Could you check a few things on this model? Use its own coordinates, in mm. Face numbers are marked on the shaded views. A direction names the side the tool comes from. Give positions to 0.01 mm unless a question says otherwise; leave off trailing zeros. Loops run counter-clockwise (first coordinate to the right, second up) from the corner with the lowest first, then second, coordinate; pieces in that order, holes last. Notation, with made-up numbers: (19.5, -4) - (35.5, -4) arc R14 cw to (35.5, 23) - close; hole circle Ø9 at (-12, 76.25). An arc over 180 degrees is marked (long way). Write each question's results on one line, items separated by ' | '. Start each with the question number.
1) I want a section at D-D, the plane z = 0. Write out the boundary of the cut face in (x, y), and give its area (3 significant figures).
2) On a 3-axis mill with a long thin cutter (end or side, diameter ignored), from which of +Z, -Z, +X, -X, +Y, -Y can I reach the whole of each face in a straight line? I mean the marked faces 4, 5 and 6. Say none if no direction works.
3) I'm going to push flat-ended pins straight in: pin 1 (5.5 mm diameter, centred on y = 53, z = -11, fed in from -X); pin 2 (1.5 mm diameter, centred on y = 7.5, z = -11.5, fed in from +X); pin 3 (6 mm diameter, centred on y = 36.5, z = -9.5, fed in from +X); pin 4 (3 mm diameter, centred on x = 0, z = 0, fed in from +Y). Where does each tip first touch, or does it pass through?
4) I want a section at B-B, the plane y = 5.5. Write out the boundary of the cut face in (x, z).
5) If I drill on probe 1 along X at (y, z) = (2.1, 0); probe 2 along Z at (x, y) = (-5, 30.5); probe 3 along Y at (x, z) = (-7, 8.5), over which ranges is the centre line in solid material (lowest first)? Write a range as [from, to].
6) I want a section at C-C, the plane x = -1.5. Write out the boundary of the cut face in (y, z), and give its area (3 significant figures).
7) If we mould it in two halves opening along Z, with no side actions, what happens to the marked faces 1, 2 and 3? For each: +Z half, -Z half, draft (parallel to the pull), parting line (faces both ways), or undercut.
8) I want a section at A-A, the plane z = 6. Write out the boundary of the cut face in (x, y).
from build123d import *

# Parameters (mm, degrees)
SKETCH1_W           = 40
SKETCH1_H           = 26
BOSS_EXTRUDE1_DEPTH = 3
SKETCH2_R           = 1.75
CUT_EXTRUDE1_DEPTH  = 3
SKETCH3_W           = 19.25
SKETCH3_H           = 3
BOSS_EXTRUDE2_DEPTH = 56.5
SKETCH5_W           = 19.25
SKETCH5_H           = 5
BOSS_EXTRUDE4_DEPTH = 12
SKETCH6_R           = 2.5
CUT_EXTRUDE2_DEPTH  = 15
SKETCH7_W           = 26
SKETCH7_H           = 60
BOSS_EXTRUDE5_DEPTH = 4


with BuildPart() as part:
    # Sketch1 → Boss-Extrude1 (new body)
    with BuildSketch(Plane(origin=(0, 0, 0), x_dir=(1, 0, 0), z_dir=(0, 1, 0))):
        Rectangle(SKETCH1_W, SKETCH1_H)
    extrude(amount=BOSS_EXTRUDE1_DEPTH)

    # Sketch2 → Cut-Extrude1 (cut)
    with BuildSketch(Plane(origin=(0, 3, 0), x_dir=(1, 0, 0), z_dir=(0, 1, 0))):
        with Locations(Location((14.3, 0, 0), (0, 0, 270))):
            Circle(SKETCH2_R)
        with Locations(Location((-14.3, 0, 0), (0, 0, 90))):
            Circle(SKETCH2_R)
    extrude(amount=-CUT_EXTRUDE1_DEPTH, mode=Mode.SUBTRACT)

    # Sketch3 → Boss-Extrude2 (add)
    with BuildSketch(Plane(origin=(0, 3, 0), x_dir=(1, 0, 0), z_dir=(0, 1, 0))):
        with Locations((0.625, -11.5)):
            Rectangle(SKETCH3_W, SKETCH3_H)
        with Locations((0.625, 11.5)):
            Rectangle(SKETCH3_W, SKETCH3_H)
    extrude(amount=BOSS_EXTRUDE2_DEPTH)

    # Sketch5 → Boss-Extrude4 (add)
    with BuildSketch(Plane(origin=(0, 59.5, 0), x_dir=(1, 0, 0), z_dir=(0, 1, 0))):
        with Locations((0.625, 10.5)):
            Rectangle(SKETCH5_W, SKETCH5_H)
        with Locations((0.625, -10.5)):
            Rectangle(SKETCH5_W, SKETCH5_H)
    extrude(amount=BOSS_EXTRUDE4_DEPTH)

    # Sketch6 → Cut-Extrude2 (cut)
    with BuildSketch(Plane(origin=(0, 3, 0), x_dir=(1, 0, 0), z_dir=(0, 1, 0))):
        with Locations(Location((0, 0, 0), (0, 0, 270))):
            Circle(SKETCH6_R)
    extrude(amount=-CUT_EXTRUDE2_DEPTH, mode=Mode.SUBTRACT)

    # Sketch7 → Boss-Extrude5 (add)
    with BuildSketch(Plane(origin=(10.25, 0, 0), x_dir=(0, 0, -1), z_dir=(1, 0, 0))):
        with Locations((0, 41.5)):
            Rectangle(SKETCH7_W, SKETCH7_H)
    extrude(amount=BOSS_EXTRUDE5_DEPTH)


solid = part.part
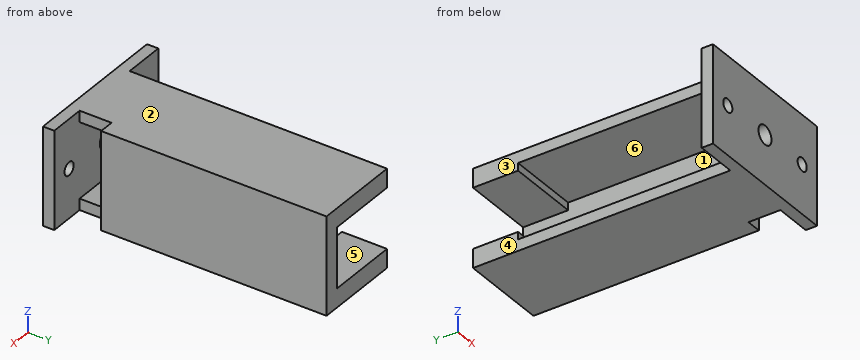
Answers:
1) outline: (-20, 0) - (-16.05, 0) - (-16.05, 3) - (-20, 3) - close; (-12.55, 0) - (-2.5, 0) - (-2.5, 3) - (-12.55, 3) - close; (2.5, 0) - (12.55, 0) - (12.55, 3) - (2.5, 3) - close; (10.25, 11.5) - (14.25, 11.5) - (14.25, 71.5) - (10.25, 71.5) - close; (16.05, 0) - (20, 0) - (20, 3) - (16.05, 3) - close | area: 324 mm2
2) face 4: +Z, -Z, -X, +Y | face 5: -X, +Y | face 6: -X
3) pin 1: stops at x = -9 | pin 2: stops at x = 10.25 | pin 3: stops at x = 14.25 | pin 4: passes through
4) outline: (-9, -13) - (10.25, -13) - (10.25, -10) - (-9, -10) - close; (-9, 10) - (10.25, 10) - (10.25, 13) - (-9, 13) - close
5) probe 1: x = [-20, -16.05], [-12.55, -2.5], [2.5, 12.55], [16.05, 20] | probe 2: z = [-13, -10], [10, 13] | probe 3: y = [0, 3], [59.5, 71.5]
6) outline: (0, -13) - (71.5, -13) - (71.5, -8) - (59.5, -8) - (59.5, -10) - (3, -10) - (3, -2) - (0, -2) - close; (0, 2) - (3, 2) - (3, 10) - (59.5, 10) - (59.5, 8) - (71.5, 8) - (71.5, 13) - (0, 13) - close | area: 525 mm2
7) face 1: undercut | face 2: +Z half | face 3: draft
8) outline: (-20, 0) - (20, 0) - (20, 3) - (-20, 3) - close; (10.25, 11.5) - (14.25, 11.5) - (14.25, 71.5) - (10.25, 71.5) - close
